Verification items for the finished model (mm, model axes). A direction names the side the tool comes from. Give positions to 0.01 mm unless a question says otherwise; leave off trailing zeros. Loops run counter-clockwise (first coordinate to the right, second up) from the corner with the lowest first, then second, coordinate; pieces in that order, holes last. Notation, with made-up numbers: (75, 71) - (88, 71) arc R14 cw to (88, 78) - close; hole circle Ø5 at (-11.75, 17). An arc over 180 degrees is marked (long way). One line per question, with ' | ' between items. Start each with the question number.
1. Depth check by flat-ended pin: pin 1 Ø12 at (y, z) = (150, 100) entering from -X; pin 2 Ø1.5 at (x, z) = (902.5, 72) entering from +Y. Enter the tip coordinate at first touch or a pass-through.
2. Section check B-B, the plane y = 190.5. Enter the section's corners in (x, z), then the cut area to 3 significant figures.
3. Mould release check, pull along Z, two halves, no side actions. Record for faces 1 (the face through (9.86, 155.38, 108.43)), 2 (the face through (1030.14, 249.976, 102.199)), 3 (the face through (513, -30, 99)), 4 (the face through (1029.86, 155.38, 108.43)): +Z half, -Z half, draft (parallel to the pull), parting line (faces both ways), or undercut.
4. Section check C-C, the plane z = 161. Enter the section's corners in (x, y).
5. Tool access check on faces 5 (the face through (441, -13, 0)), 6 (the face through (513, 0, 99)). Record the directions out of +Z, -Z, +X, -X, +Y, -Y that give a thin tool (end or side, any length) a straight path to the whole face; none if there is none.
6. Section check A-A, the plane z = 100. Enter the section's corners in (x, y), then the cut area to 3 significant figures.
7. Section check D-D, the plane x = 550. Enter the section's corners in (y, z).
8. Thickness scan on line 1 along Y through (x, z) = (1027.5, 100); line 2 along X through (y, z) = (49, 127.5); line 3 along Z through (x, y) = (7.75, 150). Record the ranges inside material, lowest first. Write a range as from..to.
from build123d import *

# Parameters (mm, degrees)
SKETCH1_W               = 1040
SKETCH1_H               = 30
BOSS_EXTRUDE1_DEPTH     = 200
BOSS_EXTRUDE3_DEPTH     = 20
CUT_EXTRUDE1_DEPTH      = 1070.065012055
CUT_EXTRUDE1_DEPTH_BACK = 1070.065012055
SKETCH3_R               = 10


with BuildPart() as part:
    # Sketch1 → Boss-Extrude1 (new body)
    with BuildSketch(Plane.XY):
        with Locations((520, -15)):
            Rectangle(SKETCH1_W, SKETCH1_H)
    extrude(amount=BOSS_EXTRUDE1_DEPTH)

    # Sketch2 → Boss-Extrude3 (add)
    with BuildSketch(Plane(origin=(1040, 0, 0), x_dir=(0, 0, -1), z_dir=(1, 0, 0))):
        with BuildLine():
            Line((-200, 0), (-200, 150))
            ThreePointArc((-200, 150), (-100, 250), (0, 150))
            Line((0, 150), (0, 0))
            Line((0, 0), (-200, 0))
        make_face()
    boss_extrude3 = extrude(amount=-BOSS_EXTRUDE3_DEPTH)

    # Mirror2: Boss-Extrude3 across plane
    add(boss_extrude3.mirror(Plane(origin=(520, 0, 0), x_dir=(0, 0, 1), z_dir=(1, 0, 0))))

    # Sketch3 → Cut-Extrude1 (cut, two sides: drawn at the far end of the back side and taken through both)
    with BuildSketch(Plane(origin=(20, 0, 0), x_dir=(0, 0, -1), z_dir=(1, 0, 0)).offset(-CUT_EXTRUDE1_DEPTH_BACK)):
        with Locations(Location((-100, 150, 0), (0, 0, 90))):
            Circle(SKETCH3_R)
    extrude(amount=CUT_EXTRUDE1_DEPTH + CUT_EXTRUDE1_DEPTH_BACK, mode=Mode.SUBTRACT)


solid = part.part
Results list:
1) pin 1: through | pin 2: y = 0
2) outline: (0, 8.57) - (20, 8.57) - (20, 191.43) - (0, 191.43) - close; (1020, 8.57) - (1040, 8.57) - (1040, 191.43) - (1020, 191.43) - close | area: 7,310 mm²
3) face 1: undercut | face 2: parting line | face 3: draft | face 4: undercut
4) outline: (0, -30) - (1040, -30) - (1040, 229.24) - (1020, 229.24) - (1020, 0) - (20, 0) - (20, 229.24) - (0, 229.24) - close
5) face 5: -Z, +X, -X, +Y, -Y | face 6: +Z, -Z, +Y
6) outline: (0, -30) - (1040, -30) - (1040, 140) - (1020, 140) - (1020, 0) - (20, 0) - (20, 140) - (0, 140) - close; (0, 160) - (20, 160) - (20, 250) - (0, 250) - close; (1020, 160) - (1040, 160) - (1040, 250) - (1020, 250) - close | area: 40,400 mm²
7) outline: (-30, 0) - (0, 0) - (0, 200) - (-30, 200) - close
8) line 1: -30..140, 160..250 | line 2: 0..20, 1020..1040 | line 3: 0..90, 110..200
